```python
from build123d import *

# Parameters (mm, degrees)
ESQUISSE1_R        = 1.03
ESQUISSE1_R_2      = 5
ESQUISSE1_W        = 5.9
ESQUISSE1_H        = 7.9
BOSS_EXTRU_1_DEPTH = 6


with BuildPart() as part:
    # Esquisse1 → Boss.-Extru.1 (new body)
    with BuildSketch(Plane.XY):
        Polygon((0, 0), (0, 49.95), (70, 49.95), (70, 6), (65.05, 6), (65.05, 0), (60, 0), (60, 6), (55.05, 6), (55.05, 0), (50, 0), (50, 6), (45.05, 6), (45.05, 0), (40, 0), (40, 6), (35.05, 6), (35.05, 0), (30, 0), (30, 6), (25.05, 6), (25.05, 0), (20, 0), (20, 6), (15.05, 6), (15.05, 0), (10, 0), (10, 6), (5.05, 6), (5.05, 0), align=None)
        with Locations((25, 36.7)):
            Circle(ESQUISSE1_R, mode=Mode.SUBTRACT)
        with Locations((45, 36.7)):
            Circle(ESQUISSE1_R, mode=Mode.SUBTRACT)
        with Locations((25, 16.7)):
            Circle(ESQUISSE1_R, mode=Mode.SUBTRACT)
        with Locations((45, 16.7)):
            Circle(ESQUISSE1_R, mode=Mode.SUBTRACT)
        with Locations((35, 26.7)):
            Circle(ESQUISSE1_R_2, mode=Mode.SUBTRACT)
        with Locations((7.5, 32)):
            Rectangle(ESQUISSE1_W, ESQUISSE1_H, mode=Mode.SUBTRACT)
        with Locations((62.5, 32)):
            Rectangle(ESQUISSE1_W, ESQUISSE1_H, mode=Mode.SUBTRACT)
    extrude(amount=BOSS_EXTRU_1_DEPTH)


solid = part.part
```
The listing builds one solid part. Answer for the finished solid, in the listing's coordinates (mm). A direction names the side the tool comes from. Give positions to 0.01 mm unless a question says otherwise; leave off trailing zeros. Order: outer loops, then holes, each group sorted by start corner. A loop starts at its lowest first (then second) coordinate and runs counter-clockwise, first axis right, second up. Notation, with made-up numbers: (35, 11) -> (92, 11) arc R21 ccw to (92, 27) -> close; hole circle Ø2 at (-16, 50). An arc over 180 degrees is marked (long way). One line per item, written item: value.
1) A tool of negligible diameter and unlimited length cuts with its end or side. For faces 4 (the flat face through (45.05, 3, 3)), 5 (the cylindrical face through (25.5, 35.8, 3)), 6 (the flat face through (68, 6, 3)), from which of +Z, -Z, +X, -X, +Y, -Y can it reach the whole face along a straight path? Write none if from no direction.
Reported:
face 4: +Z, -Z, -Y
face 5: +Z, -Z
face 6: +Z, -Z, +X, -Y
2) Find section C-C, the plane y = 26.7. Determine the outline of the cut face in (x, z).
Reported:
outline: (0, 0) -> (30, 0) -> (30, 6) -> (0, 6) -> close; (40, 0) -> (70, 0) -> (70, 6) -> (40, 6) -> close
3) Flat-ended cylindrical pins translate along their axes: P1, Ø2.5, axis at x = 27, z = 2, coming from the -Y side; P2, Ø1.8, axis at y = 3.5, z = 3, coming from the +X side; P3, Ø6, axis at x = 35, y = 26.7, coming from the -Z side. Find the tip coordinate at first contact, or state that the pin passes through.
Reported:
P1: stops at y = 6
P2: stops at x = 65.05
P3: passes through
4) Find section B-B, the plane x = 63.5. Determine the outline of the cut face in (y, z).
Reported:
outline: (0, 0) -> (28.05, 0) -> (28.05, 6) -> (0, 6) -> close; (35.95, 0) -> (49.95, 0) -> (49.95, 6) -> (35.95, 6) -> close
5) Find section A-A, the plane y = 36.7. Determine the outline of the cut face in (x, z).
Reported:
outline: (0, 0) -> (23.97, 0) -> (23.97, 6) -> (0, 6) -> close; (26.03, 0) -> (43.97, 0) -> (43.97, 6) -> (26.03, 6) -> close; (46.03, 0) -> (70, 0) -> (70, 6) -> (46.03, 6) -> close
6) Find section D-D, the plane z = 1.85. Count the separate pieces of the cut face and the enclosed holes in it, plus the area to 3 significant figures.
Reported:
separate pieces: 1
enclosed holes: 7
area: 3,100 mm^2
7) Find the intervals of material crossed by line 1 (Y direction, x = 45, z = 1.9); line 2 (Y direction, x = 61.5, z = 2.2); line 3 (Y direction, x = 16, z = 2.5), in increasing order.
Reported:
line 1: y = 0 to 15.67, 17.73 to 35.67, 37.73 to 49.95
line 2: y = 0 to 28.05, 35.95 to 49.95
line 3: y = 6 to 49.95
8) Determine the mould class of faces 1 (the flat face through (65.05, 3, 3)), 2 (the flat face through (58, 6, 3)), 3 (the flat face through (63, 0, 3)) for opening direction X: pulls with the +X half, pulls with the -X half, needs draft (parallel to the pull), parting line crosses it, or undercut.
Reported:
face 1: pulls with the +X half
face 2: undercut
face 3: needs draft
